Geometry check sheet. Reference: the model listing, model coordinates, mm. Face numbers are marked on the shaded views. A direction names the side the tool comes from. Coordinates: 2 decimals unless noted, no trailing zeros. Order: outer loops, then holes, each group sorted by start corner. A loop starts at its lowest first (then second) coordinate and runs counter-clockwise, first axis right, second up. Notation, with made-up numbers: M 1.5,-20.75 L 39.5,-20.75 A17 ccw 39.5,8.25 Z; hole C -35,-40 d2. An arc over 180 degrees is marked long. One line per item, written item: value. Start each with the question number.
1) Thickness scan on L1, parallel to Y at x = 0, z = -160; L2, parallel to X at y = -15.5, z = -18.5; L3, parallel to Y at x = 16, z = -44. Record the ranges inside material, lowest first. Write a range as from..to.
2) Sectioned sample at D-D, the plane z = -57.5. Enter the section's corners in (x, y).
3) Sectioned sample at C-C, the plane z = -156. Enter the section's corners in (x, y).
4) Draft check along Y on the marked faces 1, 2 and 3. Enter one of: pulls with the +Y half, pulls with the -Y half, needs draft (parallel to the pull), parting line crosses it, or undercut.
5) Sectioned sample at A-A, the plane y = 0. Enter the section's corners in (x, z).
6) Go/stop test with flat-tipped pins: P1, Ø3, axis at y = 28.5, z = -43, coming from the +X side; P2, Ø10, axis at x = 50.5, z = -55.5, coming from the -Y side; P3, Ø6, axis at y = 20, z = -42, coming from the -X side. Record where each tip stops, or that it passes through.
7) Access from +Z, -Z, +X, -X, +Y, -Y to the whole of each face (thin tool, end or side, straight path). Record for the marked faces 4 and 5.
```python
from build123d import *


with BuildPart() as part:
    # Sketch1 → Revolve1 (revolve)
    with BuildSketch(Plane(origin=(0, 0, 0), x_dir=(1, 0, 0), z_dir=(0, 1, 0)), mode=Mode.PRIVATE) as revolve1_sk:
        with BuildLine():
            Line((44, 3), (47, 3))
            ThreePointArc((47, 3), (49.121320344, 2.121320344), (50, 0))
            Line((50, 0), (70, 0))
            Line((70, 0), (70, 20))
            Line((70, 20), (56.475570251, 20))
            ThreePointArc((56.475570251, 20), (55.158468064, 20.494927966), (54.493236583, 21.734758171))
            Line((54.493236583, 21.734758171), (38, 145))
            Line((38, 145), (38, 185))
            Line((38, 185), (25, 185))
            Line((25, 185), (25, 145))
            Line((25, 145), (44, 3))
        make_face()
    revolve(revolve1_sk.sketch.rotate(Axis((0, 0, -195.705477905), (0, 0, 1)), 180), axis=Axis((0, 0, -195.705477905), (0, 0, 1)))


solid = part.part
```
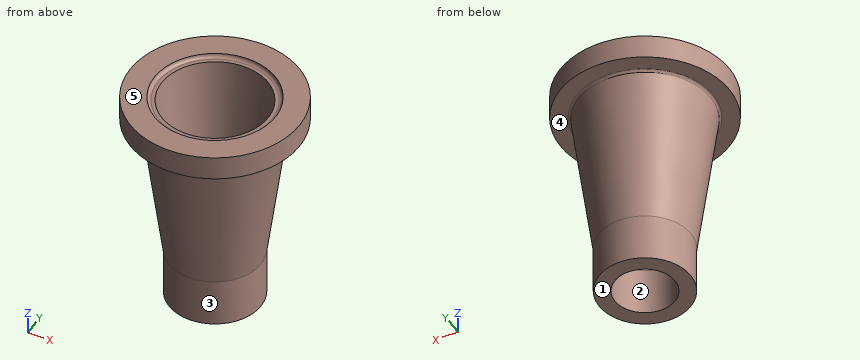
Final values:
1. L1: y = -38..-25, 25..38
1. L2: x = -68.26..-38.96, 38.96..68.26
1. L3: y = -48.97..-35.03, 35.03..48.97
2. outline: C 0,0 d99.42; hole C 0,0 d73.42
3. outline: C 0,0 d76; hole C 0,0 d50
4. face 1: needs draft
4. face 2: undercut
4. face 3: parting line crosses it
5. outline: M -70,-20 L -56.48,-20 A2 cw -54.49,-21.73 L -38,-145 L -38,-185 L -25,-185 L -25,-145 L -44,-3 L -47,-3 A3 cw -50,0 L -70,0 Z; M 25,-185 L 38,-185 L 38,-145 L 54.49,-21.73 A2 cw 56.48,-20 L 70,-20 L 70,0 L 50,0 A3 cw 47,-3 L 44,-3 L 25,-145 Z
6. P1: stops at x = 44.06
6. P2: stops at y = -20.79
6. P3: stops at x = -48.99
7. face 4: -Z
7. face 5: +Z, +X, -X, +Y, -Y
